```python
from build123d import *

# Parameters (mm, degrees)
BOSS_EXTRUDE1_DEPTH      = 1.5
BOSS_EXTRUDE2_DEPTH      = 6
BOSS_EXTRUDE2_DEPTH_BACK = 3


with BuildPart() as part:
    # Sketch1 → Boss-Extrude1 (new body)
    with BuildSketch(Plane(origin=(0, 0, 0), x_dir=(1, 0, 0), z_dir=(0, 1, 0))):
        Polygon((-0.635, 1.27), (0.635, 1.27), (1.27, 0.635), (1.27, -0.635), (0.635, -1.27), (1.27, -1.905), (1.27, -3.175), (0.635, -3.81), (1.27, -4.445), (1.27, -5.715), (0.635, -6.35), (1.27, -6.985), (1.27, -8.255), (0.635, -8.89), (1.27, -9.525), (1.27, -10.795), (0.635, -11.43), (-0.635, -11.43), (-1.27, -10.795), (-1.27, -9.525), (-0.635, -8.89), (-1.27, -8.255), (-1.27, -6.985), (-0.635, -6.35), (-1.27, -5.715), (-1.27, -4.445), (-0.635, -3.81), (-1.27, -3.175), (-1.27, -1.905), (-0.635, -1.27), (-1.27, -0.635), (-1.27, 0.635), align=None)
    extrude(amount=BOSS_EXTRUDE1_DEPTH)

    # Sketch2 → Boss-Extrude2 (add, two sides: drawn at the far end of the back side and taken through both)
    with BuildSketch(Plane(origin=(0, 1.5, 0), x_dir=(1, 0, 0), z_dir=(0, 1, 0)).offset(-BOSS_EXTRUDE2_DEPTH_BACK)):
        Polygon((0.5, 0.375), (0.375, 0.5), (-0.375, 0.5), (-0.5, 0.375), (-0.5, -0.375), (-0.375, -0.5), (0.375, -0.5), (0.5, -0.375), align=None)
        Polygon((0.5, -2.165), (0.375, -2.04), (-0.375, -2.04), (-0.5, -2.165), (-0.5, -2.915), (-0.375, -3.04), (0.375, -3.04), (0.5, -2.915), align=None)
        Polygon((0.5, -4.705), (0.375, -4.58), (-0.375, -4.58), (-0.5, -4.705), (-0.5, -5.455), (-0.375, -5.58), (0.375, -5.58), (0.5, -5.455), align=None)
        Polygon((0.5, -7.245), (0.375, -7.12), (-0.375, -7.12), (-0.5, -7.245), (-0.5, -7.995), (-0.375, -8.12), (0.375, -8.12), (0.5, -7.995), align=None)
        Polygon((0.5, -9.785), (0.375, -9.66), (-0.375, -9.66), (-0.5, -9.785), (-0.5, -10.535), (-0.375, -10.66), (0.375, -10.66), (0.5, -10.535), align=None)
    extrude(amount=BOSS_EXTRUDE2_DEPTH + BOSS_EXTRUDE2_DEPTH_BACK)


solid = part.part
```
Source: CAD feature listing. Evaluate the final solid. Frame: model axes, mm. Give positions to 0.01 mm unless a question says otherwise; leave off trailing zeros. Loops run counter-clockwise (first coordinate to the right, second up) from the corner with the lowest first, then second, coordinate; pieces in that order, holes last. Notation, with made-up numbers: (-30, 36) - (-21, 36) arc R13 cw to (-21, 54) - close; hole circle Ø4 at (62.25, 87.5). An arc over 180 degrees is marked (long way). Use CSV: the item, a comma, the result in double quotes. Start each with the question number.
1. Pin query (flat end, axial travel): pin 1 (0.8 mm diameter, centred on y = -0.5, z = 2.5, fed in from -X); pin 2 (0.6 mm diameter, centred on x = 0, y = 3.5, fed in from +Z); pin 3 (0.6 mm diameter, centred on x = 0, y = -1, fed in from -Z). Return the tip coordinate at first contact, or that it passes through.
2. Ray query, L1, parallel to Z at x = 0, y = 4; L2, parallel to Z at x = -0.4, y = 4.75 (3 decimals); L3, parallel to Y at x = -0.65, z = 3.5. Return the intervals inside material, ascending.
3. Section B-B (y = 6.25). Count the separate pieces of the cut face and the enclosed holes in it, then the cut area to 3 significant figures.
4. Section C-C (z = 1). Output: boundary loops of the cut face in (x, y) (3 decimals).
5. Section A-A (z = 7.5). Output: boundary loops of the cut face in (x, y).
Response:
1,pin 1,"x = -0.5"
1,pin 2,"z = 10.66"
1,pin 3,"z = -0.5"
2,L1,"-0.5 to 0.5, 2.04 to 3.04, 4.58 to 5.58, 7.12 to 8.12, 9.66 to 10.66"
2,L2,"-0.475 to 0.475, 2.065 to 3.015, 4.605 to 5.555, 7.145 to 8.095, 9.685 to 10.635"
2,L3,"0 to 1.5"
3,separate pieces,"5"
3,enclosed holes,"0"
3,area,"4.84 mm²"
4,outline,"(-0.905, 0) - (0.905, 0) - (0.905, 1.5) - (-0.905, 1.5) - close"
5,outline,"(-1.27, 0) - (-0.5, 0) - (-0.5, -1.5) - (0.5, -1.5) - (0.5, 0) - (1.27, 0) - (1.27, 1.5) - (0.5, 1.5) - (0.5, 7.5) - (-0.5, 7.5) - (-0.5, 1.5) - (-1.27, 1.5) - close"
